```python
from build123d import *

# Parameters (mm, degrees)
SKETCH1_W           = 60
SKETCH1_H           = 30
BOSS_EXTRUDE1_DEPTH = 5
SKETCH2_R           = 1.65
CUT_EXTRUDE1_DEPTH  = 34.911649916
SKETCH3_W           = 60
SKETCH3_H           = 5
BOSS_EXTRUDE2_DEPTH = 20
SKETCH4_R           = 1.65
CUT_EXTRUDE2_DEPTH  = 10
FILLET1_R           = 10
CHAMFER1_SIZE       = 0.6


with BuildPart() as part:
    # Sketch1 → Boss-Extrude1 (new body)
    with BuildSketch(Plane(origin=(0, 0, 0), x_dir=(1, 0, 0), z_dir=(0, 1, 0))):
        Rectangle(SKETCH1_W, SKETCH1_H)
    extrude(amount=BOSS_EXTRUDE1_DEPTH)

    # Sketch2 → Cut-Extrude1 (cut, through all)
    with BuildSketch(Plane(origin=(0, 5, 0), x_dir=(1, 0, 0), z_dir=(0, 1, 0))):
        with Locations(Location((-22.5, 7.5, 0), (0, 0, 270))):
            Circle(SKETCH2_R)
        with Locations(Location((22.5, 7.5, 0), (0, 0, 270))):
            Circle(SKETCH2_R)
    extrude(amount=-CUT_EXTRUDE1_DEPTH, mode=Mode.SUBTRACT)

    # Sketch3 → Boss-Extrude2 (add)
    with BuildSketch(Plane.XZ):
        with Locations((0, 12.5)):
            Rectangle(SKETCH3_W, SKETCH3_H)
    extrude(amount=BOSS_EXTRUDE2_DEPTH)

    # Sketch4 → Cut-Extrude2 (cut)
    with BuildSketch(Plane(origin=(0, 0, 10), x_dir=(-1, 0, 0), z_dir=(0, 0, -1))):
        with Locations((-12, -10)):
            Circle(SKETCH4_R)
        with Locations((12, -10)):
            Circle(SKETCH4_R)
    extrude(amount=-CUT_EXTRUDE2_DEPTH, mode=Mode.SUBTRACT)

    # Fillet1
    fillet1_edges = [part.edges().sort_by_distance(p)[0] for p in [
        (-30, -20, 12.5),
        (30, -20, 12.5),
        (-30, 2.5, -15),
        (30, 2.5, -15),
    ]]
    fillet(fillet1_edges, radius=FILLET1_R)

    # Chamfer1
    chamfer1_edges = [part.edges().sort_by_distance(p)[0] for p in [
        (0, 5, 15),
        (30, 0, 2.5),
        (0, -20, 10),
        (0, -20, 15),
        (30, -5, 10),
        (-30, -5, 10),
        (27.071067812, -17.071067812, 10),
        (-27.071067812, -17.071067812, 10),
        (30, 5, 5),
        (-30, 0, 2.5),
        (-30, 5, 5),
        (27.071067812, -17.071067812, 15),
        (-27.071067812, -17.071067812, 15),
        (0, 0, -15),
        (27.071067812, 0, -12.071067812),
        (-27.071067812, 0, -12.071067812),
        (0, 5, -15),
        (27.071067812, 5, -12.071067812),
        (-27.071067812, 5, -12.071067812),
        (30, -2.5, 15),
        (-30, -2.5, 15),
    ]]
    chamfer(chamfer1_edges, length=CHAMFER1_SIZE)


solid = part.part
```
Input: part model. Units: mm. Frame: model coordinates. Coordinates: 2 decimals unless noted, no trailing zeros. Order: outer loops, then holes, each group sorted by start corner. A loop starts at its lowest first (then second) coordinate and runs counter-clockwise, first axis right, second up. Notation, with made-up numbers: (72.25, 50) - (96.25, 50) arc R7 ccw to (96.25, 55) - close; hole circle Ø7 at (68.25, 41). An arc over 180 degrees is marked (long way). Return JSON: item names as keys, results as strings.
Q1. Cut plane B-B (z = -3). Return loops of the section in (x, y).
The answers:
{"outline": "(-30, 0.6) - (-29.4, 0) - (29.4, 0) - (30, 0.6) - (30, 4.4) - (29.4, 5) - (-29.4, 5) - (-30, 4.4) - close"}
Q2. Ray query, probe 1 along Y at (x, z) = (-12, 12.45); probe 2 along Y at (x, z) = (-20, 7.5); probe 3 along Z at (x, y) = (13, -8.25). Return the intervals inside material, ascending.
The answers:
{"probe 1": "y = -20 to -11.65, -8.35 to 5", "probe 2": "y = 0 to 5", "probe 3": "z = 10 to 15"}
Q3. Cut plane C-C (x = 4). Return loops of the section in (y, z).
The answers:
{"outline": "(-20, 10.6) - (-19.4, 10) - (0, 10) - (0, -14.4) - (0.6, -15) - (4.4, -15) - (5, -14.4) - (5, 14.4) - (4.4, 15) - (-19.4, 15) - (-20, 14.4) - close"}
Q4. Draft query along X for faces 1 (the cylindrical face through (-20.864, 2.535, -7.715)), 2 (the flat face through (0, -10, 10)), 3 (the cylindrical face through (24.136, 2.535, -7.715)), 4 (the cylindrical face through (26.99, -17.15, 12.53)). Return one class per face: +X half, -X half, draft (parallel to the pull), parting line (faces both ways), or undercut.
The answers:
{"face 1": "undercut", "face 2": "draft", "face 3": "undercut", "face 4": "+X half"}
Q5. Cut plane A-A (x = 12). Return loops of the section in (y, z).
The answers:
{"outline": "(-20, 10.6) - (-19.4, 10) - (-11.65, 10) - (-11.65, 15) - (-19.4, 15) - (-20, 14.4) - close; (-8.35, 10) - (0, 10) - (0, -14.4) - (0.6, -15) - (4.4, -15) - (5, -14.4) - (5, 14.4) - (4.4, 15) - (-8.35, 15) - close"}
Q6. Cut plane D-D (z = -7.5). State how many separate pieces and enclosed holes the cut face has, then the cut area to 3 significant figures.
The answers:
{"separate pieces": "3", "enclosed holes": "0", "area": "263 mm2"}
Q7. First-contact query: pin 1 (3 mm diameter, centred on x = 12.5, z = -7.5, fed in from -Y); pin 2 (5.5 mm diameter, centred on x = 12, y = -10, fed in from -Z); pin 3 (1.5 mm diameter, centred on y = -3.5, z = 9.5, fed in from +X); pin 4 (2.5 mm diameter, centred on x = -22.5, z = -7.5, fed in from +Y). Flat tips, straight axial feed; report the tip coordinate or a pass-through.
The answers:
{"pin 1": "stops at y = 0", "pin 2": "stops at z = 10", "pin 3": "stops at x = 29.65", "pin 4": "passes through"}
